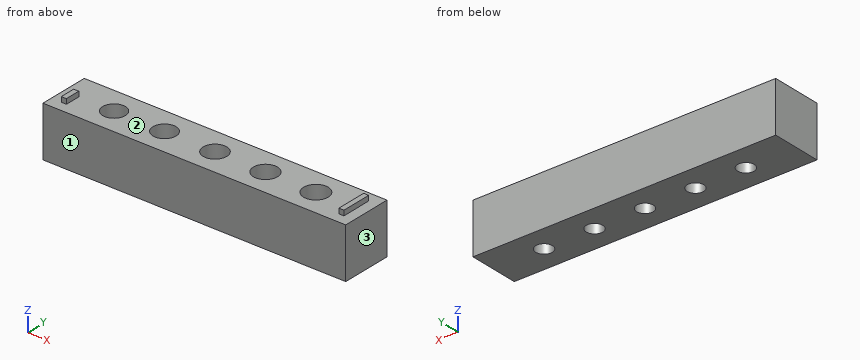
```python
from build123d import *

# Parameters (mm, degrees)
SKETCH_W      = 60
SKETCH_H      = 10
SKETCH_R      = 1.65
PAD_DEPTH     = 10
SKETCH001_W   = 1
SKETCH001_H   = 3
SKETCH001_H_2 = 6
PAD001_DEPTH  = 1
SKETCH002_R   = 2.25
SKETCH002_R_2 = 2.3
SKETCH002_R_3 = 2.35
SKETCH002_R_4 = 2.4
SKETCH002_R_5 = 2.45
POCKET_DEPTH  = 5


with BuildPart() as part:
    # Sketch → Pad (new body)
    with BuildSketch(Plane.XY):
        Rectangle(SKETCH_W, SKETCH_H)
        with Locations((-20, 0)):
            Circle(SKETCH_R, mode=Mode.SUBTRACT)
        with Locations((-10, 0)):
            Circle(SKETCH_R, mode=Mode.SUBTRACT)
        Circle(SKETCH_R, mode=Mode.SUBTRACT)
        with Locations((10, 0)):
            Circle(SKETCH_R, mode=Mode.SUBTRACT)
        with Locations((20, 0)):
            Circle(SKETCH_R, mode=Mode.SUBTRACT)
    extrude(amount=PAD_DEPTH)

    # Sketch001 → Pad001 (join)
    with BuildSketch(Plane.XY.offset(10)):
        with Locations((-27.5, -1.5)):
            Rectangle(SKETCH001_W, SKETCH001_H)
        with Locations((27.5, 0)):
            Rectangle(SKETCH001_W, SKETCH001_H_2)
    extrude(amount=PAD001_DEPTH)

    # Sketch002 (on Face11 of Pad) → Pocket (cut)
    with BuildSketch(Plane.XY.offset(10)):
        with Locations((-20, 0)):
            Circle(SKETCH002_R)
        with Locations((-10, 0)):
            Circle(SKETCH002_R_2)
        Circle(SKETCH002_R_3)
        with Locations((10, 0)):
            Circle(SKETCH002_R_4)
        with Locations((20, 0)):
            Circle(SKETCH002_R_5)
    extrude(amount=-POCKET_DEPTH, mode=Mode.SUBTRACT)


solid = part.part
```
The model under review builds one solid part; all positions refer to its coordinate system, in mm. Face numbers are marked on the shaded views. Give positions to 0.01 mm unless a question says otherwise; leave off trailing zeros. Write each loop counter-clockwise with the first axis right and the second up, starting at its lowest first coordinate (ties: lowest second). Pieces come first, ordered by that corner, then holes. Notation, with made-up numbers: (4.25, 58) -> (40.25, 58) arc R13 ccw to (40.25, 62) -> close; hole circle Ø9 at (14, 10.5). An arc over 180 degrees is marked (long way). Answer in a Markdown table with one row per item.
1) Mouldability with a two-part tool opening along X and no side actions: class the marked faces 1, 2 and 3 as +X half, -X half, draft (parallel to the pull), parting line (faces both ways), or undercut.
Worked answers:
| item | result |
|---|---|
| face 1 | draft |
| face 2 | undercut |
| face 3 | +X half |
2) Add section A-A on x = -20. State the section outline as (y, z) points.
Worked answers:
| item | result |
|---|---|
| outline | (-5, 0) -> (-1.65, 0) -> (-1.65, 5) -> (-2.25, 5) -> (-2.25, 10) -> (-5, 10) -> close; (1.65, 0) -> (5, 0) -> (5, 10) -> (2.25, 10) -> (2.25, 5) -> (1.65, 5) -> close |
3) For L1, parallel to X at y = 0, z = 2.25; L2, parallel to Y at x = -20, z = 1.25; L3, parallel to Y at x = 10, z = 8, list the stretches that pass through material, from the lowest coordinate up. Write a range as [from, to].
Worked answers:
| item | result |
|---|---|
| L1 | [-30, -21.65], [-18.35, -11.65], [-8.35, -1.65], [1.65, 8.35], [11.65, 18.35], [21.65, 30] |
| L2 | [-5, -1.65], [1.65, 5] |
| L3 | [-5, -2.4], [2.4, 5] |
4) Add section D-D on z = 3.5. State the section outline as (x, y) points, plus the area to 3 significant figures.
Worked answers:
| item | result |
|---|---|
| outline | (-30, -5) -> (30, -5) -> (30, 5) -> (-30, 5) -> close; hole circle Ø3.3 at (-20, 0); hole circle Ø3.3 at (-10, 0); hole circle Ø3.3 at (0, 0); hole circle Ø3.3 at (10, 0); hole circle Ø3.3 at (20, 0) |
| area | 557 mm² |
5) Add section C-C on x = 10. State the section outline as (y, z) points, plus the area to 3 significant figures.
Worked answers:
| item | result |
|---|---|
| outline | (-5, 0) -> (-1.65, 0) -> (-1.65, 5) -> (-2.4, 5) -> (-2.4, 10) -> (-5, 10) -> close; (1.65, 0) -> (5, 0) -> (5, 10) -> (2.4, 10) -> (2.4, 5) -> (1.65, 5) -> close |
| area | 59.5 mm² |
6) Clearance check with flat-ended pins moving along their axes: P1, Ø2, axis at x = -7, y = 3.5, coming from the +Z side; P2, Ø0.5, axis at x = 27.5, z = 10.5, coming from the -Y side; P3, Ø1.4, axis at x = 0, y = 0, coming from the +Z side; P4, Ø0.8, axis at y = 0, z = 10.5, coming from the +X side. State where each tip first meets the part, or that it passes through.
Worked answers:
| item | result |
|---|---|
| P1 | z = 10 |
| P2 | y = -3 |
| P3 | through |
| P4 | x = 28 |
7) Add section B-B on z = 6. State the section outline as (x, y) points, plus the area to 3 significant figures.
Worked answers:
| item | result |
|---|---|
| outline | (-30, -5) -> (30, -5) -> (30, 5) -> (-30, 5) -> close; hole circle Ø4.5 at (-20, 0); hole circle Ø4.6 at (-10, 0); hole circle Ø4.7 at (0, 0); hole circle Ø4.8 at (10, 0); hole circle Ø4.9 at (20, 0) |
| area | 513 mm² |
